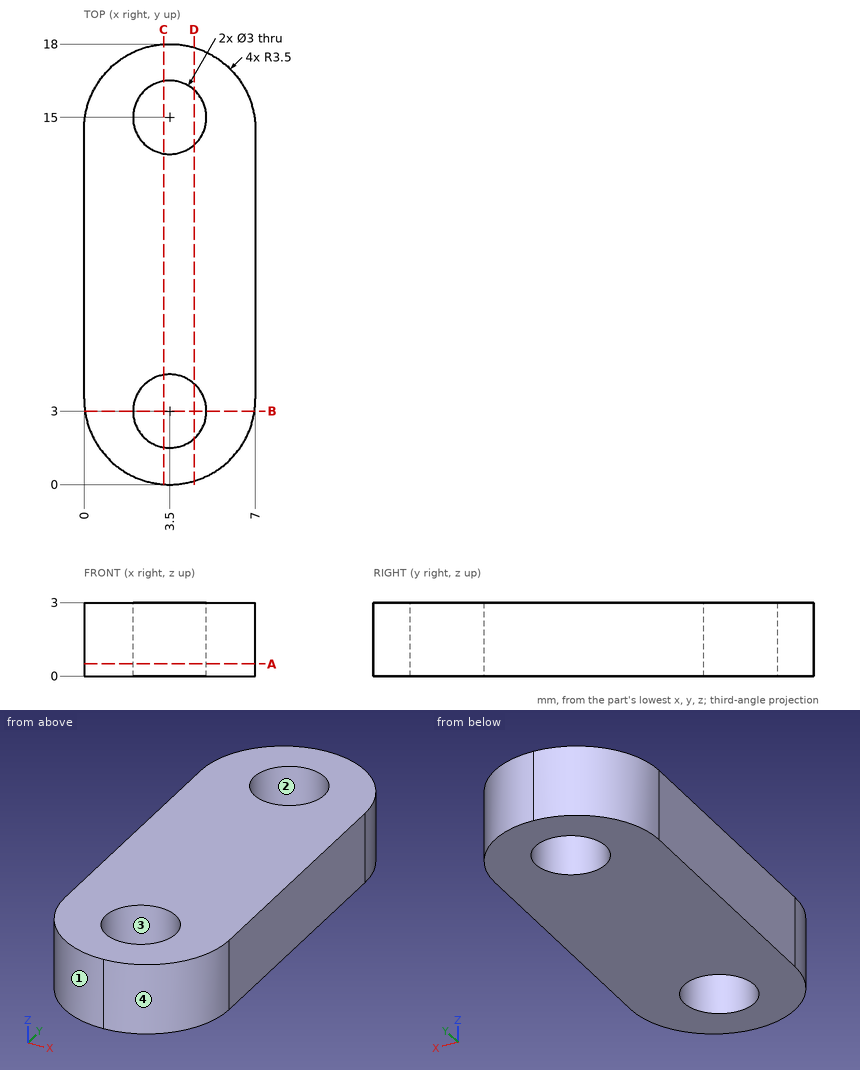
Verification items for this drawing (mm, ordinates from the low corner). Give positions to 0.01 mm unless a question says otherwise; leave off trailing zeros. Loops run counter-clockwise (first coordinate to the right, second up) from the corner with the lowest first, then second, coordinate; pieces in that order, holes last. Notation, with made-up numbers: M -34,4 L -13,4 A31 ccw -13,31 Z; hole C -16,4.25 d10. An arc over 180 degrees is marked long. Answer in a Markdown table with one row per item.
1) Cross-section at C-C (x = 3.25). Enter the section's corners in (y, z).
Solutions:
| item | result |
|---|---|
| outline | M 0.01,0 L 1.52,0 L 1.52,3 L 0.01,3 Z; M 4.48,0 L 13.52,0 L 13.52,3 L 4.48,3 Z; M 16.48,0 L 17.99,0 L 17.99,3 L 16.48,3 Z |
2) Cross-section at B-B (y = 3). Enter the section's corners in (x, z).
Solutions:
| item | result |
|---|---|
| outline | M 0.04,0 L 2,0 L 2,3 L 0.04,3 Z; M 5,0 L 6.96,0 L 6.96,3 L 5,3 Z |
3) Cross-section at D-D (x = 4.5). Enter the section's corners in (y, z).
Solutions:
| item | result |
|---|---|
| outline | M 0.15,0 L 1.88,0 L 1.88,3 L 0.15,3 Z; M 4.12,0 L 13.88,0 L 13.88,3 L 4.12,3 Z; M 16.12,0 L 17.85,0 L 17.85,3 L 16.12,3 Z |
4) Cross-section at A-A (z = 0.5). Count the separate pieces of the cut face and the enclosed holes in it, plus the area to 3 significant figures.
Solutions:
| item | result |
|---|---|
| separate pieces | 1 |
| enclosed holes | 2 |
| area | 101 mm^2 |
5) Depth check by flat-ended pin: pin 1 (2 mm diameter, centred on x = 2.5, y = 3, fed in from -Z); pin 2 (1.5 mm diameter, centred on x = 5.5, z = 1, fed in from +Y). Enter the tip coordinate at first touch or a pass-through.
Solutions:
| item | result |
|---|---|
| pin 1 | stops at z = 0 |
| pin 2 | stops at y = 17.77 |
6) Mould release check, pull along X, two halves, no side actions. Record for the marked faces 1, 2, 3 and 4: released by +X, released by -X, zero draft, split by the parting line, or undercut.
Solutions:
| item | result |
|---|---|
| face 1 | released by -X |
| face 2 | undercut |
| face 3 | undercut |
| face 4 | released by +X |
7) Thickness scan on line 1 (Y direction, x = 3.5, z = 1.4); line 2 (Y direction, x = 4.75, z = 0.85); line 3 (X direction, y = 15, z = 2.1) (1 decimal). Record the ranges inside material, lowest first.
Solutions:
| item | result |
|---|---|
| line 1 | y = 0 to 1.5, 4.5 to 13.5, 16.5 to 18 |
| line 2 | y = 0.23 to 2.17, 3.83 to 14.17, 15.83 to 17.77 |
| line 3 | x = 0 to 2, 5 to 7 |
